```python
from build123d import *

# Parameters (mm, degrees)
F3_DEPTH = 5
F4_R     = 4
F5_DEPTH = 10


with BuildPart() as f1:
    # F0 (on Front) → F1 (revolve)
    with BuildSketch(Plane.XZ):
        Polygon((10, 30), (-40, 30), (-40, 0), (0, 0), (0, 8), align=None)
    revolve(axis=Axis((-2.905972, 0, 0), (1, 0, 0)))

    # F2 (on face) → F3 (cut)
    with BuildSketch(Plane.YZ):
        Polygon((0, -6.928203), (6, -3.464102), (6, 3.464102), (0, 6.928203), (-6, 3.464102), (-6, -3.464102), align=None)
    extrude(amount=-F3_DEPTH, mode=Mode.SUBTRACT)

    # F4 (on face) → F5 (join)
    with BuildSketch(Plane(origin=(-40, 0, 0), x_dir=(0, -1, 0), z_dir=(-1, 0, 0))):
        Circle(F4_R)
    extrude(amount=F5_DEPTH)


solid = f1.part
```
Build history of the part. All positions in model axes, mm. A direction names the side the tool comes from. Give positions to 0.01 mm unless a question says otherwise; leave off trailing zeros. Loops run counter-clockwise (first coordinate to the right, second up) from the corner with the lowest first, then second, coordinate; pieces in that order, holes last.
1) Band-saw the part on B-B on x = -41.5. List the corners of the cut face in (y, z), then the cut area to 3 significant figures.
Values follow:
outline: circle Ø8 at (0, 0)
area: 50.3 mm2
2) 3-axis set-ups, long thin cutter, end or side, ignore diameter. For faces 1 (the face through (-15.35, -1.32, -29.97)), 2 (the face through (-2, -6, 0)): which of +Z, -Z, +X, -X, +Y, -Y reach the whole face in a straight line?
Values follow:
face 1: +X, -X
face 2: +X
3) Band-saw the part on D-D on x = -28. List the corners of the cut face in (y, z), then the cut area to 3 significant figures.
Values follow:
outline: circle Ø60 at (0, 0)
area: 2,830 mm2
4) Drop flat-ended pins along their axis: P1, Ø1.5, axis at x = -2.5, z = -0.5, coming from the -Y side; P2, Ø2, axis at y = 17, z = -20.5, coming from the -X side; P3, Ø6, axis at y = -4.5, z = -1.5, coming from the +X side. Give the stop position or say it passes through.
Values follow:
P1: stops at y = -30
P2: stops at x = -40
P3: stops at x = 0
5) Band-saw the part on C-C on x = 1.5. List the corners of the cut face in (y, z).
Values follow:
outline: circle Ø60 at (0, 0); hole circle Ø22.6 at (0, 0)
6) Two-plate mould, pull along Y, no slides. Class faces 3 (the face through (0.626, 9.153, -2.033)), 4 (the face through (-50, 0, 0)), 5 (the face through (-44.93, 0.867, -3.905)): released by +Y, released by -Y, zero draft, split by the parting line, or undercut.
Values follow:
face 3: undercut
face 4: zero draft
face 5: split by the parting line
7) Band-saw the part on A-A on z = 0. List the corners of the cut face in (x, y).
Values follow:
outline: (-50, -4) - (-40, -4) - (-40, -30) - (10, -30) - (0, -8) - (0, -6) - (-5, -6) - (-5, 6) - (0, 6) - (0, 8) - (10, 30) - (-40, 30) - (-40, 4) - (-50, 4) - close
8) Probe line 1 along Y through (x, z) = (-0.5, -1); line 2 along Z through (x, y) = (7.5, -1); line 3 along X through (y, z) = (5, 16). List the from-to ranges inside material, lowest first.
Values follow:
line 1: y = -29.98 to -6, 6 to 29.98
line 2: z = -29.98 to -24.48, 24.48 to 29.98
line 3: x = -40 to 3.98
